Check sheet for the modelled part. Datum: model origin and axes. Units: mm. Coordinates: 2 decimals unless noted, no trailing zeros. Order: outer loops, then holes, each group sorted by start corner. A loop starts at its lowest first (then second) coordinate and runs counter-clockwise, first axis right, second up. Notation, with made-up numbers: (-2.75, -5) -> (45.25, -5) arc R34 ccw to (45.25, 26) -> close; hole circle Ø4 at (-8.5, 34.25). An arc over 180 degrees is marked (long way). Put each result on its own line as item: value. Start each with the question number.
Autodesk Inventor part; units mm, degrees
ref_plane "YZ Plane" through (0, 0, 0) normal (1, 0, 0) x (0, 1, 0)
ref_plane "XZ Plane" through (0, 0, 0) normal (0, 1, 0) x (-1, 0, 0)
ref_plane "XY Plane" through (0, 0, 0) normal (0, 0, 1) x (1, 0, 0)
sketch "Szkic1" plane through (0, 0, 0) normal (1, 0, 0) x (0, 1, 0)
  line L0 (0, 0) -> (6, 0)
  line L1 (6, 0) -> (6, -178)
  line L2 (6, -178) -> (0, -178)
  line L3 (0, -178) -> (0, 0)
  line L4 (0, -89) -> (100, -89)
  line L5 (100, -129.3113) -> (100, -149)
  line L6 (100, -149) -> (6, -149)
  line L7 (100, -48.6887) -> (100, -29)
  line L8 (100, -29) -> (6, -29)
  line L9 (100, -89) -> (80, -89)
  arc A0 (100, -48.6887) -> (100, -129.3113) centre (80, -89) ccw
  line L10 (80, -40) -> (80, -138)
  point P0 (6, -29)
  dimension "d0" = 6
  dimension "d1" = 178
  dimension "d2" = 100
  dimension "d3" = 60
  dimension "d4" = 20
  dimension "d5" = 90
  dimension "d6" = 98
extrude "Wyciągnięcie proste1" add sketch "Szkic1" against normal blind 6 contours L0 L1 L4 L3 | L4 L1 L2 L3 | L8 L7 A0 L4 L1 | L4 A0 L5 L6 L1
hole "Otwór1" at (0, 80, -40) at (0, 80, -138) direction (-1, 0, 0) diameter 6.2 depth 33 tip angle 118
pattern_circular "Szyk kołowy1" count 4 over 360 about axis through (0, 80, -89) along (-1, 0, 0) of "Otwór1"
fillet "Zaokrąglenie1" radius 2 2 edges at (-3, 100, -29) (-3, 100, -149)
extrude "Wyciągnięcie proste3" cut sketch "Szkic1" against normal blind 37.25 contours L0 L1 L4 L3 | L4 L1 L2 L3
properties part number "łapa1"
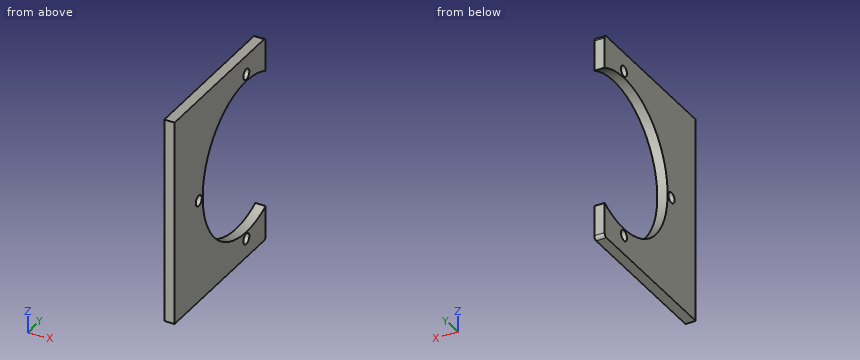
1) Sectioned sample at C-C (x = -5). Record the boundary of the cut face in (y, z), plus the area to 3 significant figures.
2) Sectioned sample at A-A (y = 31). Record the boundary of the cut face in (x, z), plus the area to 3 significant figures.
3) Sectioned sample at B-B (z = -40). Record the boundary of the cut face in (x, y), plus the area to 3 significant figures.
4) Sectioned sample at D-D (y = 80). Record the boundary of the cut face in (x, z).
5) Scan lines: line 1 along Z through (x, y) = (-2.35, 80); line 2 along Z through (x, y) = (-1.7, 31); line 3 along Y through (x, z) = (-3.45, -138). Record each from-to range of solid material in increasing order. Write a range as [from, to].
6) Gauge pin test, flat end, axial feed: pin 1 (5.5 mm diameter, centred on y = 31, z = -89, fed in from -X). Record the tip position at first contact, or that the pin passes through.
Entries:
1. outline: (6, -149) -> (98, -149) arc R2 ccw to (100, -147) -> (100, -129.31) arc R45 cw (long way) to (100, -48.69) -> (100, -31) arc R2 ccw to (98, -29) -> (6, -29) -> close; hole circle Ø6.2 at (31, -89); hole circle Ø6.2 at (80, -138); hole circle Ø6.2 at (80, -40)
1. area: 6,270 mm2
2. outline: (-6, -149) -> (0, -149) -> (0, -92.1) -> (-6, -92.1) -> close; (-6, -85.9) -> (0, -85.9) -> (0, -29) -> (-6, -29) -> close
2. area: 683 mm2
3. outline: (-6, 6) -> (0, 6) -> (0, 76.9) -> (-6, 76.9) -> close; (-6, 83.1) -> (0, 83.1) -> (0, 100) -> (-6, 100) -> close
3. area: 527 mm2
4. outline: (-6, -149) -> (0, -149) -> (0, -141.1) -> (-6, -141.1) -> close; (-6, -134.9) -> (0, -134.9) -> (0, -134) -> (-6, -134) -> close; (-6, -44) -> (0, -44) -> (0, -43.1) -> (-6, -43.1) -> close; (-6, -36.9) -> (0, -36.9) -> (0, -29) -> (-6, -29) -> close
5. line 1: z = [-149, -141.1], [-134.9, -134], [-44, -43.1], [-36.9, -29]
5. line 2: z = [-149, -92.1], [-85.9, -29]
5. line 3: y = [6, 76.9], [83.1, 100]
6. pin 1: passes through
